from build123d import *

# Parameters (mm, degrees)
F0_W           = 25.4
F0_H           = 25.4
F1_DEPTH       = 19.05
F3_DEPTH       = 19.051
F3_DEPTH_BACK  = 25.4
F5_DEPTH       = 25.4
F5_DEPTH_BACK  = 6.35
F6_W           = 12.7
F6_H           = 12.7
F7_DEPTH       = 25.401
F8_W           = 6.35
F8_H           = 6.35
F9_DEPTH       = 4.7625
F11_DEPTH      = 25.4
F11_DEPTH_BACK = 6.35


with BuildPart() as f1:
    # F0 (on Front) → F1 (new body, symmetric)
    with BuildSketch(Plane.XZ):
        with Locations((-12.7, 12.7)):
            Rectangle(F0_W, F0_H)
    extrude(amount=F1_DEPTH, both=True)

    # F2 (on Front) → F3 (cut, two sides)
    with BuildSketch(Plane.XZ) as f3_sk:
        Polygon((-25.4, 25.4), (0, 6.35), (0, 25.4), align=None)
    extrude(amount=-F3_DEPTH, mode=Mode.SUBTRACT)
    extrude(f3_sk.sketch, amount=F3_DEPTH_BACK, mode=Mode.SUBTRACT)

    # F4 (on Front) → F5 (cut, two sides)
    with BuildSketch(Plane.XZ) as f5_sk:
        Polygon((-25.4, 25.4), (-25.4, 19.05), (-16.9333333333, 19.05), align=None)
    extrude(amount=F5_DEPTH, mode=Mode.SUBTRACT)
    extrude(f5_sk.sketch, amount=-F5_DEPTH_BACK, mode=Mode.SUBTRACT)

    # F6 (on Right) → F7 (cut, through all)
    with BuildSketch(Plane.YZ):
        with Locations((-12.7, 12.7)):
            Rectangle(F6_W, F6_H)
    extrude(amount=-F7_DEPTH, mode=Mode.SUBTRACT)

    # F8 (on Right) → F9 (cut, symmetric)
    with BuildSketch(Plane.YZ):
        with Locations((3.175, 9.525)):
            Rectangle(F8_W, F8_H)
    extrude(amount=F9_DEPTH, both=True, mode=Mode.SUBTRACT)

    # F10 (on Front) → F11 (cut, two sides)
    with BuildSketch(Plane.XZ) as f11_sk:
        Polygon((0, 6.35), (-9.525, 13.49375), (-9.525, 6.35), align=None)
    extrude(amount=F11_DEPTH, mode=Mode.SUBTRACT)
    extrude(f11_sk.sketch, amount=-F11_DEPTH_BACK, mode=Mode.SUBTRACT)


solid = f1.part
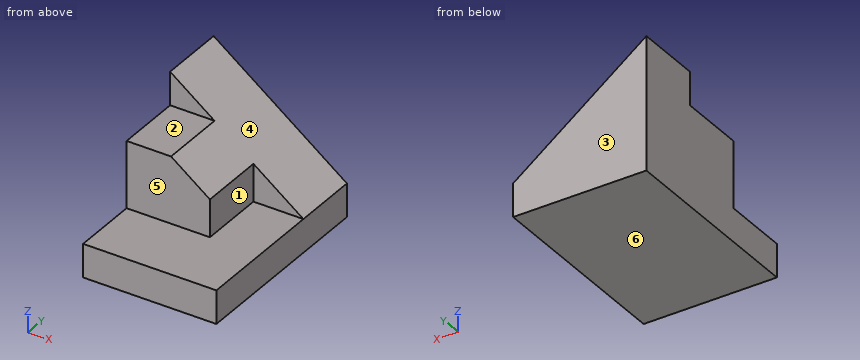
Could you check a few things on this model? Use its own coordinates, in mm. Face numbers are marked on the shaded views. A direction names the side the tool comes from. Give positions to 0.01 mm unless a question says otherwise; leave off trailing zeros. Order: outer loops, then holes, each group sorted by start corner. A loop starts at its lowest first (then second) coordinate and runs counter-clockwise, first axis right, second up.
1. Thinking about a two-plate mould opening in Z: for the marked faces 4, 5 and 6, which applies, +Z half, -Z half, draft (parallel to the pull), parting line (faces both ways), or undercut?
Answers below:
face 4: +Z half
face 5: draft
face 6: -Z half
2. Suppose I cut it at D-D (x = -5). Write out the boundary of the cut face in (y, z).
Answers below:
outline: (-19.05, 0) - (19.05, 0) - (19.05, 10.1) - (6.35, 10.1) - (6.35, 6.35) - (-19.05, 6.35) - close
3. I need wall thicknesses on L1, parallel to Y at x = -15, z = 8.5; L2, parallel to Z at x = -9, y = -6; L3, parallel to Y at x = -6.5, z = 9. Which ranges of each line are inside material? Lowest first, please.
Answers below:
L1: y = -6.35 to 19.05
L2: z = 0 to 6.35
L3: y = 6.35 to 19.05
4. Which directions (+Z, -Z, +X, -X, +Y, -Y) give clear straight access to the entire face, cutting with the end or side of a thin tool? Please do the marked faces 1, 2 and 3.
Answers below:
face 1: +Z, +X, -Y
face 2: +Z, +X, -X, -Y
face 3: +Z, -Z, +X, -X, +Y
5. Suppose I cut it at C-C (z = 7.25). Write out the boundary of the cut face in (x, y) (3 decimals), plus the area to 3 significant figures.
Answers below:
outline: (-25.4, -6.35) - (-9.525, -6.35) - (-9.525, 6.35) - (-1.2, 6.35) - (-1.2, 19.05) - (-25.4, 19.05) - close
area: 509 mm2
6. Suppose I cut it at B-B (y = -3). Write out the boundary of the cut face in (x, z) (3 decimals), plus the area to 3 significant figures.
Answers below:
outline: (-25.4, 0) - (0, 0) - (0, 6.35) - (-9.525, 6.35) - (-9.525, 13.494) - (-16.933, 19.05) - (-25.4, 19.05) - close
area: 342 mm2
7. Suppose I cut it at A-A (x = -18). Write out the boundary of the cut face in (y, z).
Answers below:
outline: (-19.05, 0) - (19.05, 0) - (19.05, 19.85) - (6.35, 19.85) - (6.35, 19.05) - (-6.35, 19.05) - (-6.35, 6.35) - (-19.05, 6.35) - close
8. For pin 1 (12 mm diameter, centred on x = -13.5, y = -2, fed in from +Z); pin 2 (1.5 mm diameter, centred on x = -3.5, z = 10.5, fed in from -Y); pin 3 (4 mm diameter, centred on x = -21.5, y = 14.5, fed in from +Z) (3 decimals); pin 4 (5.5 mm diameter, centred on x = -6.5, z = 9.5, fed in from -Y), each with a flat end and sliding along its axis, tell me the tip position at first contact or that it passes through.
Answers below:
pin 1: stops at z = 19.05
pin 2: passes through
pin 3: stops at z = 23.975
pin 4: stops at y = 6.35
